Verification items for the finished model (mm, model axes). A direction names the side the tool comes from. Give positions to 0.01 mm unless a question says otherwise; leave off trailing zeros. Write each loop counter-clockwise with the first axis right and the second up, starting at its lowest first coordinate (ties: lowest second). Pieces come first, ordered by that corner, then holes. Notation, with made-up numbers: (7, 39.25) -> (59, 39.25) arc R17 ccw to (59, 47.25) -> close; hole circle Ø9 at (-14.75, 17.25). An arc over 180 degrees is marked (long way). Use one line per item in the form item = value. Start each with the question number.
(1) Depth check by flat-ended pin: pin 1 Ø4 at (y, z) = (29, 8) entering from -X; pin 2 Ø4.5 at (x, y) = (29.36, 52.39) entering from -Z; pin 3 Ø5.5 at (x, y) = (-2.5, -26.5) entering from +Z (3 decimals); pin 4 Ø1.4 at (y, z) = (10.5, 6.5) entering from +X. Enter the tip coordinate at first touch or a pass-through.
(2) Release check for a two-part mould opening along Y. For faces 1 (the face through (47.67, 73, 7.31)), 2 (the face through (28, -1, 9.525)), 3 (the face through (32.407, -50.593, -5.146)) record: pulls with the +Y half, pulls with the -Y half, needs draft (parallel to the pull), parting line crosses it, or undercut.
(3) Section check A-A, the plane y = 11.5. Record the cut outline in (x, z) (1 decimal).
(4) Scan lines: L1, parallel to X at y = -50.8, z = 4.5; L2, parallel to X at y = -51, z = -0.5; L3, parallel to X at y = -50.8, z = 6.5. Record each from-to range of solid material in increasing order.
(5) Set-up check for faces 4 (the face through (0, -1, 3.175)), 5 (the face through (-47.6, 73.07, 7.31)): record each of +Z, -Z, +X, -X, +Y, -Y from which the full face is reachable in a straight line by a thin tool's end or side.
(6) Section check B-B, the plane x = 6. Record the cut outline in (y, z) (3 decimals), plus the area to 3 significant figures.
from build123d import *

# Parameters (mm, degrees)
F0_W     = 101.6
F0_H     = 19.05
F1_DEPTH = 76.2
F3_D     = 7.9375
F3_DEPTH = 12.7
F3_TIP   = 2.3846655818
F5_DEPTH = 152.401
F7_D     = 5.1054
F8_SIZE  = 5.08
F9_R     = 5.08


with BuildPart() as f1:
    # F0 (on Front) → F1 (new body, symmetric)
    with BuildSketch(Plane.XZ):
        Rectangle(F0_W, F0_H)
    extrude(amount=F1_DEPTH, both=True)

    # F3
    with Locations(Plane.XY.offset(9.525)):
        with Locations((-31.75, -50.8), (31.75, -50.8)):
            Hole(F3_D / 2, depth=F3_DEPTH)
            with Locations((0, 0, -(F3_DEPTH + F3_TIP / 2))):  # 118° drill point
                Cone(0, F3_D / 2, F3_TIP, mode=Mode.SUBTRACT)

    # F4 (on face) → F5 (cut, through all)
    with BuildSketch(Plane.XZ.offset(76.2)):
        with BuildLine():
            Line((10.8450762928, 9.525), (-10.8450762928, 9.525))
            Line((-10.8450762928, 9.525), (-10.8450762928, 4.7625))
            ThreePointArc((-10.8450762928, 4.7625), (-10.3801083079, 3.6399679849), (-9.2575762928, 3.175))
            Line((-9.2575762928, 3.175), (9.2575762928, 3.175))
            ThreePointArc((9.2575762928, 3.175), (10.3801083079, 3.6399679849), (10.8450762928, 4.7625))
            Line((10.8450762928, 4.7625), (10.8450762928, 9.525))
        make_face()
    extrude(amount=-F5_DEPTH, mode=Mode.SUBTRACT)

    # F7 (through all)
    with Locations(Plane.XY.offset(9.525)):
        with Locations((-29.3624, 52.3875), (29.3624, 52.3875)):
            Hole(F7_D / 2)

    # F8
    f8_edges = [f1.edges().sort_by_distance(p)[0] for p in [
        (50.8, 76.2, 0),
        (50.8, -76.2, 0),
        (-50.8, -76.2, 0),
        (-50.8, 76.2, 0),
    ]]
    chamfer(f8_edges, length=F8_SIZE)

    # F9
    f9_edges = [f1.edges().sort_by_distance(p)[0] for p in [
        (-48.26, 73.66, 9.525),
        (-28.282538, 76.2, 9.525),
        (-48.26, -73.66, 9.525),
        (48.26, -73.66, 9.525),
        (48.26, 73.66, 9.525),
        (50.8, 0, 9.525),
        (-50.8, 0, 9.525),
        (-28.282538, -76.2, 9.525),
        (28.282538, -76.2, 9.525),
        (28.282538, 76.2, 9.525),
    ]]
    fillet(f9_edges, radius=F9_R)


solid = f1.part
Completed:
q1.pin_1 = -50.56
q1.pin_2 = through
q1.pin_3 = 3.175
q1.pin_4 = 50.62
q2.face_1 = pulls with the +Y half
q2.face_2 = needs draft
q2.face_3 = undercut
q3.outline = (-50.8, -9.5) -> (50.8, -9.5) -> (50.8, 4.4) arc R5.1 ccw to (45.7, 9.5) -> (10.8, 9.5) -> (10.8, 4.8) arc R1.6 cw to (9.3, 3.2) -> (-9.3, 3.2) arc R1.6 cw to (-10.8, 4.8) -> (-10.8, 9.5) -> (-45.7, 9.5) arc R5.1 ccw to (-50.8, 4.4) -> close
q4.L1 = -50.8 to -35.72, -27.78 to -10.82, 10.82 to 27.78, 35.72 to 50.8
q4.L2 = -50.8 to -35.71, -27.79 to 27.79, 35.71 to 50.8
q4.L3 = -50.37 to -35.72, -27.78 to -10.85, 10.85 to 27.78, 35.72 to 50.37
q5.face_4 = +Z, +Y, -Y
q5.face_5 = +Z, -X, +Y
q6.outline = (-76.2, -9.525) -> (76.2, -9.525) -> (76.2, 3.175) -> (-76.2, 3.175) -> close
q6.area = 1,940 mm²
